Check sheet for the modelled part. Datum: model origin and axes. Units: mm. Give positions to 0.01 mm unless a question says otherwise; leave off trailing zeros. Loops run counter-clockwise (first coordinate to the right, second up) from the corner with the lowest first, then second, coordinate; pieces in that order, holes last. Notation, with made-up numbers: M 81.5,46 L 106.5,46 A12 ccw 106.5,55 Z; hole C 1.5,-30 d9. An arc over 180 degrees is marked long. Write each question's results on one line, items separated by ' | '. Start each with the question number.
1. Sectioned sample at D-D on y = 445.5. Record the cut outline in (x, z).
2. Draft check along Y on faces 1 (the flat face through (115, 347, -5)), 2 (the flat face through (-95.18, 561.45, -2.46)), 3 (the cylindrical face through (12.37, 67.33, -2.46)). Enter one of: pulls with the +Y half, pulls with the -Y half, needs draft (parallel to the pull), parting line crosses it, or undercut.
3. Sectioned sample at C-C on y = 636. Record the cut outline in (x, z), and give its area (3 significant figures).
4. Sectioned sample at A-A on y = 47.5. Record the cut outline in (x, z), and give its area (3 significant figures).
5. Material ranges on line 1 along X through (y, z) = (780, -2.8); line 2 along Y through (x, z) = (245, -1.65); line 3 along X through (y, z) = (40.5, -3.5), recorded low to high.
6. Sectioned sample at B-B on z = -3.2. Give the number of separate pieces and of enclosed holes in the cut face, and give its area (3 significant figures).
7. Go/stop test with flat-tipped pins: pin 1 (5.5 mm diameter, centred on x = 134.98, y = 33, fed in from +Z); pin 2 (10 mm diameter, centred on x = 80.5, y = 670, fed in from +Z); pin 3 (1 mm diameter, centred on y = 536, z = -2, fed in from -X). Record where each tip stops, or that it passes through.
```python
from build123d import *

# Parameters (mm, degrees)
BASE_FLANGE1_DEPTH         = 5
FILLET1_R                  = 20
F_10_0_10_DIAMETER_HOLE1_D = 10
SKETCH10_R                 = 20
CUT_EXTRUDE1_DEPTH         = 964.833217765
M10_CLEARANCE_HOLE3_D      = 11
M8_CLEARANCE_HOLE1_D       = 9


# Sheet-metal steps are written as plain solids
with BuildPart() as part:
    # Sketch1 → Base-Flange1 (new body)
    with BuildSketch(Plane.XY):
        Polygon((0, 0), (400, 0), (400, 800), (252.239031103, 800), (131.200331365, 884.752209972), (-327.660817716, 229.43057454), align=None)
    extrude(amount=-BASE_FLANGE1_DEPTH)

    # Fillet1
    fillet1_edges = [part.edges().sort_by_distance(p)[0] for p in [
        (-327.660817716, 229.43057454, -2.5),
        (131.200331365, 884.752209972, -2.5),
        (252.239031103, 800, -2.5),
        (400, 800, -2.5),
        (400, 0, -2.5),
        (0, 0, -2.5),
    ]]
    fillet(fillet1_edges, radius=FILLET1_R)

    # Ø10.0 (10) Diameter Hole1 (through all)
    with Locations(Plane.XY):
        with Locations((245.933055326, 780), (136.111843524, 856.897640359), (380, 780)):
            Hole(F_10_0_10_DIAMETER_HOLE1_D / 2)

    # Sketch10 → Cut-Extrude1 (cut, through all)
    with BuildSketch(Plane.XY):
        with Locations((14.976692472, 47.5)):
            Circle(SKETCH10_R)
    extrude(amount=-CUT_EXTRUDE1_DEPTH, mode=Mode.SUBTRACT)

    # M10 Clearance Hole3 (through all)
    with Locations(Plane.XY):
        with Locations((-23.994450699, 70), (53.947835642, 25)):
            Hole(M10_CLEARANCE_HOLE3_D / 2)

    # M8 Clearance Hole1 (through all)
    with Locations(Plane.XY):
        with Locations((-124.404492942, 127.394525174), (-78.518378033, 192.926688717), (-45.752296262, 169.983631263), (-91.63841117, 104.45146772), (-101.461435488, 160.160606946), (-68.695353716, 137.217549491), (134.976692472, 113), (174.976692472, 33), (134.976692472, 33), (174.976692472, 113), (134.976692472, 73), (174.976692472, 73)):
            Hole(M8_CLEARANCE_HOLE1_D / 2)


solid = part.part
```
Output values:
1) outline: M -176.37,-5 L 400,-5 L 400,0 L -176.37,0 Z
2) face 1: needs draft | face 2: pulls with the +Y half | face 3: undercut
3) outline: M -42.98,-5 L 400,-5 L 400,0 L -42.98,0 Z | area: 2,210 mm2
4) outline: M -67.84,-5 L -5.02,-5 L -5.02,0 L -67.84,0 Z; M 34.98,-5 L 400,-5 L 400,0 L 34.98,0 Z | area: 2,140 mm2
5) line 1: 57.85 to 240.93, 250.93 to 375, 385 to 400 | line 2: 0 to 775.09, 784.91 to 805.07 | line 3: -57.84 to -3.76, 33.71 to 400
6) separate pieces: 1 | enclosed holes: 18 | area: 435,000 mm2
7) pin 1: through | pin 2: z = 0 | pin 3: x = -113.35
